```python
from build123d import *

# Parameters (mm, degrees)
F0_W     = 1.778
F0_H     = 5.08
F1_DEPTH = 10.16
F3_DEPTH = 1.016
F4_R     = 0.508


with BuildPart() as f1:
    # F0 (on Top) → F1 (new body)
    with BuildSketch(Plane.XY):
        Polygon((-3.302, 5.842), (-3.302, 5.08), (-1.524, 5.08), (-1.524, 8.636), (-3.302, 8.636), align=None)
        Polygon((-1.524, 5.08), (-3.302, 5.08), (-3.302, 4.572), (-3.302, 2.54), (-3.302, 0), (-1.524, 0), align=None)
        Polygon((-3.302, 4.572), (-3.302, 5.08), (-3.302, 5.842), (-5.334, 5.842), (-5.334, 4.572), align=None)
        with BuildLine():
            Line((-3.302, 2.54), (-3.302, 4.572))
            Line((-3.302, 4.572), (-5.334, 4.572))
            ThreePointArc((-5.334, 4.572), (-4.738841, 3.135159), (-3.302, 2.54))
        make_face()
        with BuildLine():
            ThreePointArc((1.524, 0), (0, -1.524), (-1.524, 0))
            Line((-1.524, 0), (-3.302, 0))
            ThreePointArc((-3.302, 0), (0, -3.302), (3.302, 0))
            Line((3.302, 0), (1.524, 0))
        make_face()
        with Locations((2.413, 2.54)):
            Rectangle(F0_W, F0_H)
        with BuildLine():
            ThreePointArc((5.08, 8.636), (2.565528, 7.594472), (1.524, 5.08))
            Line((1.524, 5.08), (3.302, 5.08))
            ThreePointArc((3.302, 5.08), (3.822764, 6.337236), (5.08, 6.858))
            Line((5.08, 6.858), (5.08, 8.636))
        make_face()
        with BuildLine():
            ThreePointArc((5.08, 6.858), (3.822764, 6.337236), (3.302, 5.08))
            Line((3.302, 5.08), (14.986, 5.08))
            Line((14.986, 5.08), (14.986, 6.858))
            Line((14.986, 6.858), (5.08, 6.858))
        make_face()
    extrude(amount=F1_DEPTH)

    # F2 (on face) → F3 (join)
    with BuildSketch(Plane(origin=(0, 8.636, 0), x_dir=(-1, 0, 0), z_dir=(0, 1, 0))):
        with BuildLine():
            Line((3.302, 6.35), (3.302, 3.81))
            ThreePointArc((3.302, 3.81), (4.572, 5.08), (3.302, 6.35))
        make_face()
    extrude(amount=-F3_DEPTH)

    # F4
    f4_edges = [f1.edges().sort_by_distance(p)[0] for p in [
        (-1.524, 8.636, 5.08),
    ]]
    fillet(f4_edges, radius=F4_R)


solid = f1.part
```
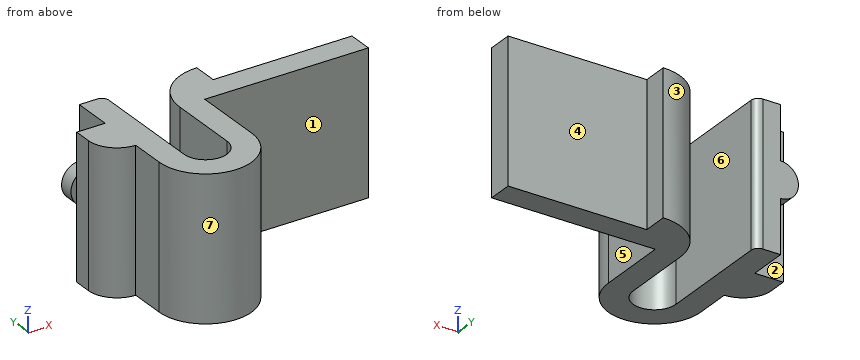
Here's how the part is built. I have some questions about the finished solid (model axes, mm). Face numbers are marked on the shaded views. A direction names the side the tool comes from. Give positions to 0.01 mm unless a question says otherwise; leave off trailing zeros. Loops run counter-clockwise (first coordinate to the right, second up) from the corner with the lowest first, then second, coordinate; pieces in that order, holes last. Notation, with made-up numbers: M 70,-30.5 L 127,-30.5 A35 ccw 127,2.5 Z; hole C 83,-29.5 d1. An arc over 180 degrees is marked long. Put each result on its own line as item: value. Start each with the question number.
(1) If we mould it in two halves opening along X, with no side actions, what happens to the marked faces 5, 6 and 7? For each: +X half, -X half, draft (parallel to the pull), parting line (faces both ways), or undercut.
(2) Will these pins go through, and if not, where does the flat tip stop? pin 1 Ø2.5 at (y, z) = (2, 4) entering from +X; pin 2 Ø5 at (y, z) = (-1, 8) entering from -X; pin 3 Ø1.4 at (y, z) = (7.5, 6) entering from -X; pin 4 Ø2 at (x, y) = (5, -0.5) entering from -Z.
(3) For the marked faces 1, 2, 3 and 4, which set-ups out of +Z, -Z, +X, -X, +Y, -Y let a thin tool reach every point of the face, with its end or its side?
(4) I want a section at C-C on y = -0.5. Please give me the cut outline in (x, z), then the cut area to 3 significant figures.
(5) I want a section at B-B on z = 5.08. Please give me the cut outline in (x, y).
(6) I want a section at D-D on x = 0. Please give me the cut outline in (y, z), then the cut area to 3 significant figures.
(7) I want a section at A-A on y = 2. Please give me the cut outline in (x, z).
(8) I need wall thicknesses on line 1 along X through (y, z) = (1.25, 2.75); line 2 along X through (y, z) = (4.75, 4.75); line 3 along Y through (x, z) = (13.5, 1.5). Which ranges of each line are inside material? Lowest first, please. Write a range as [from, to].
Answer block:
1. face 5: +X half
1. face 6: undercut
1. face 7: parting line
2. pin 1: x = 3.3
2. pin 2: x = -3.3
2. pin 3: x = -4.55
2. pin 4: through
3. face 1: +Z, -Z, +X, -Y
3. face 2: +Z, -Z, -X
3. face 3: +Z, -Z, +Y
3. face 4: +Z, -Z, +X, +Y
4. outline: M -3.26,0 L -1.44,0 L -1.44,10.16 L -3.26,10.16 Z; M 1.44,0 L 3.26,0 L 3.26,10.16 L 1.44,10.16 Z
4. area: 37.1 mm^2
5. outline: M -5.33,4.57 A2.03 ccw -3.3,2.54 L -3.3,0 A3.3 ccw 3.3,0 L 3.3,5.08 L 14.99,5.08 L 14.99,6.86 L 5.08,6.86 L 5.08,8.64 A3.56 ccw 1.52,5.08 L 1.52,0 A1.52 cw -1.52,0 L -1.52,8.13 A0.51 ccw -2.03,8.64 L -4.57,8.64 L -4.57,7.62 L -3.3,7.62 L -3.3,5.84 L -5.33,5.84 Z
6. outline: M -3.3,0 L -1.52,0 L -1.52,10.16 L -3.3,10.16 Z
6. area: 18.1 mm^2
7. outline: M -3.3,0 L -1.52,0 L -1.52,10.16 L -3.3,10.16 Z; M 1.52,0 L 3.3,0 L 3.3,10.16 L 1.52,10.16 Z
8. line 1: [-3.3, -1.52], [1.52, 3.3]
8. line 2: [-5.33, -1.52], [1.52, 3.3]
8. line 3: [5.08, 6.86]
